from build123d import *

# Parameters (mm, degrees)
BOSS_EXTRUDE1_DEPTH     = 2
SKETCH2_R               = 1.575
BOSS_EXTRUDE2_DEPTH     = 4
SKETCH3_R               = 3.5
BOSS_EXTRUDE3_DEPTH     = 1
SKETCH4_W               = 2
SKETCH4_H               = 17
BOSS_EXTRUDE4_DEPTH     = 0.001
SKETCH5_W               = 18
SKETCH5_H               = 2
BOSS_EXTRUDE5_DEPTH     = 0.001
SKETCH6_W               = 2.001
SKETCH6_H               = 2
BOSS_EXTRUDE6_DEPTH     = 5
BOSS_EXTRUDE7_DEPTH     = 0.001
CUT_EXTRUDE1_DEPTH      = 20.519323784
SKETCH9_W               = 2.937742252
SKETCH9_H               = 8
CUT_EXTRUDE2_DEPTH      = 0.001
CUT_EXTRUDE11_START     = -0.001
SKETCH21_R              = 9.75
SKETCH21_R_2            = 3.5
CUT_EXTRUDE11_DEPTH     = 0.001
SKETCH10_W              = 32
SKETCH10_H              = 2
BOSS_EXTRUDE8_DEPTH     = 7
FILLET1_R               = 0.5
SKETCH11_R              = 0.625
BOSS_EXTRUDE9_DEPTH     = 2
SKETCH14_W              = 2
SKETCH14_H              = 2
CUT_EXTRUDE5_DEPTH      = 22.401355237
SKETCH12_R              = 0.675
CUT_EXTRUDE3_DEPTH      = 2.5
CUT_EXTRUDE6_DEPTH      = 2
FILLET2_R               = 0.5
FILLET3_R               = 0.5
FILLET4_R               = 2
CUT_EXTRUDE7_DEPTH      = 26.019992106
CUT_EXTRUDE7_DEPTH_BACK = 1
SKETCH19_R              = 0.625
CUT_EXTRUDE9_DEPTH      = 2


with BuildPart() as part:
    # Sketch1 → Boss-Extrude1 (new body)
    with BuildSketch(Plane.XY):
        Polygon((-11, 6), (-11, 11), (11, 11), (11, 6), (11, -6), (-11, -6), align=None)
    extrude(amount=BOSS_EXTRUDE1_DEPTH)

    # Sketch3 → Boss-Extrude3 (add)
    with BuildSketch(Plane(origin=(0, 0, 0), x_dir=(-1, 0, 0), z_dir=(0, 0, -1))):
        with Locations(Location((0, 0, 0), (0, 0, 180))):
            Circle(SKETCH3_R)
    extrude(amount=BOSS_EXTRUDE3_DEPTH)

    # Sketch4 → Boss-Extrude4 (add)
    with BuildSketch(Plane(origin=(0, 0, 0), x_dir=(-1, 0, 0), z_dir=(0, 0, -1))):
        with Locations((10, 2.5)):
            Rectangle(SKETCH4_W, SKETCH4_H)
        with Locations((-10, 2.5)):
            Rectangle(SKETCH4_W, SKETCH4_H)
    extrude(amount=BOSS_EXTRUDE4_DEPTH)

    # Sketch5 → Boss-Extrude5 (add)
    with BuildSketch(Plane(origin=(0, 0, 0), x_dir=(-1, 0, 0), z_dir=(0, 0, -1))):
        with Locations((0, 10)):
            Rectangle(SKETCH5_W, SKETCH5_H)
    extrude(amount=BOSS_EXTRUDE5_DEPTH)

    # Sketch6 → Boss-Extrude6 (add)
    with BuildSketch(Plane(origin=(11, 0, 0), x_dir=(0, 0, -1), z_dir=(1, 0, 0))):
        with Locations((-0.9995, -5)):
            Rectangle(SKETCH6_W, SKETCH6_H)
        with Locations((-0.9995, 5)):
            Rectangle(SKETCH6_W, SKETCH6_H)
    boss_extrude6 = extrude(amount=BOSS_EXTRUDE6_DEPTH)

    # Mirror1: Boss-Extrude6 across plane
    add(boss_extrude6.mirror(Plane(origin=(0, 0, 0), x_dir=(0, 0, 1), z_dir=(1, 0, 0))))

    # Sketch7 → Boss-Extrude7 (add)
    with BuildSketch(Plane(origin=(0, 0, -0.001), x_dir=(-1, 0, 0), z_dir=(0, 0, -1))):
        with BuildLine():
            ThreePointArc((-6.708203932, -6), (-8.407551231, -3.211398808), (-9, 0))
            Line((-9, 0), (-9, -6))
            Line((-9, -6), (-6.708203932, -6))
        make_face()
        with BuildLine():
            Line((-9, 9), (-9, 0))
            ThreePointArc((-9, 0), (-6.363961031, 6.363961031), (0, 9))
            Line((0, 9), (-9, 9))
        make_face()
    boss_extrude7 = extrude(amount=-BOSS_EXTRUDE7_DEPTH)

    # Sketch8 → Cut-Extrude1 (cut, through all)
    with BuildSketch(Plane(origin=(0, 0, -0.001), x_dir=(-1, 0, 0), z_dir=(0, 0, -1))):
        with BuildLine():
            Line((-11, 4), (-9.16515139, 4))
            ThreePointArc((-9.16515139, 4), (-10, 0), (-9.16515139, -4))
            Line((-9.16515139, -4), (-11, -4))
            Line((-11, -4), (-11, 4))
        make_face()
    cut_extrude1 = extrude(amount=-CUT_EXTRUDE1_DEPTH, mode=Mode.SUBTRACT)

    # Sketch9 → Cut-Extrude2 (cut)
    with BuildSketch(Plane(origin=(0, 0, -0.001), x_dir=(-1, 0, 0), z_dir=(0, 0, -1))):
        with Locations((-9.531128874, 0)):
            Rectangle(SKETCH9_W, SKETCH9_H)
    cut_extrude2 = extrude(amount=-CUT_EXTRUDE2_DEPTH, mode=Mode.SUBTRACT)

    # Mirror2: Boss-Extrude7, Cut-Extrude1, Cut-Extrude2 across plane
    add(boss_extrude7.mirror(Plane(origin=(0, 0, 0), x_dir=(0, 0, 1), z_dir=(1, 0, 0))))
    add(cut_extrude1.mirror(Plane(origin=(0, 0, 0), x_dir=(0, 0, 1), z_dir=(1, 0, 0))), mode=Mode.SUBTRACT)
    add(cut_extrude2.mirror(Plane(origin=(0, 0, 0), x_dir=(0, 0, 1), z_dir=(1, 0, 0))), mode=Mode.SUBTRACT)

    # Sketch21 → Cut-Extrude11 (cut)
    with BuildSketch(Plane(origin=(0, 0, -0.001), x_dir=(-1, 0, 0), z_dir=(0, 0, -1)).offset(CUT_EXTRUDE11_START)):
        Circle(SKETCH21_R)
        with Locations(Location((0, 0, 0), (0, 0, 180))):
            Circle(SKETCH21_R_2, mode=Mode.SUBTRACT)
    extrude(amount=CUT_EXTRUDE11_DEPTH, mode=Mode.SUBTRACT)

    # Sketch10 → Boss-Extrude8 (add)
    with BuildSketch(Plane.XY.offset(2)):
        with Locations((0, -5)):
            Rectangle(SKETCH10_W, SKETCH10_H)
        with Locations((0, 5)):
            Rectangle(SKETCH10_W, SKETCH10_H)
    extrude(amount=BOSS_EXTRUDE8_DEPTH)

    # Fillet1
    fillet1_edges = [part.edges().sort_by_distance(p)[0] for p in [
        (10, 0, 2),
        (-10, 0, 2),
    ]]
    fillet(fillet1_edges, radius=FILLET1_R)

    # Sketch11 → Boss-Extrude9 (add)
    with BuildSketch(Plane(origin=(0, 0, -0.001), x_dir=(-1, 0, 0), z_dir=(0, 0, -1))):
        with Locations(Location((-13, -5, 0), (0, 0, 180))):
            Circle(SKETCH11_R)
    boss_extrude9 = extrude(amount=BOSS_EXTRUDE9_DEPTH)

    # Sketch14 → Cut-Extrude5 (cut, through all)
    with BuildSketch(Plane(origin=(0, 0, -0.001), x_dir=(-1, 0, 0), z_dir=(0, 0, -1))):
        with Locations((10, 7)):
            Rectangle(SKETCH14_W, SKETCH14_H)
        with Locations((-10, 7)):
            Rectangle(SKETCH14_W, SKETCH14_H)
    extrude(amount=-CUT_EXTRUDE5_DEPTH, mode=Mode.SUBTRACT)

    # Sketch12 → Cut-Extrude3 (cut)
    with BuildSketch(Plane(origin=(0, 0, -0.001), x_dir=(-1, 0, 0), z_dir=(0, 0, -1))):
        with Locations((13, -5)):
            Circle(SKETCH12_R)
    cut_extrude3 = extrude(amount=-CUT_EXTRUDE3_DEPTH, mode=Mode.SUBTRACT)

    # Sketch16 → Cut-Extrude6 (cut)
    with BuildSketch(Plane(origin=(0, 6, 0), x_dir=(1, 0, 0), z_dir=(0, 1, 0))):
        with BuildLine():
            Line((-9, -1), (-9, -2))
            ThreePointArc((-9, -2), (-8.75, -1.5), (-9, -1))
        make_face()
    cut_extrude6 = extrude(amount=CUT_EXTRUDE6_DEPTH, mode=Mode.SUBTRACT)

    # Mirror3: Boss-Extrude9, Cut-Extrude3 across plane
    add(boss_extrude9.mirror(Plane.ZX))
    add(cut_extrude3.mirror(Plane.ZX), mode=Mode.SUBTRACT)

    # Mirror4: Cut-Extrude6 across plane
    add(cut_extrude6.mirror(Plane(origin=(0, 0, 0), x_dir=(0, 0, 1), z_dir=(1, 0, 0))), mode=Mode.SUBTRACT)

    # Fillet2
    fillet2_edges = [part.edges().sort_by_distance(p)[0] for p in [
        (12.375, -5, -0.001),
        (12.375, 5, -0.001),
    ]]
    fillet(fillet2_edges, radius=FILLET2_R)

    # Fillet3
    # the kernel refuses this fillet: 0.5 mm, written as the material it takes off along each edge
    with BuildSketch(Plane(origin=(-13, -5, -0.001), x_dir=(-1, 0, 0), z_dir=(0, -1, 0))) as fillet3_piece_1:
        with BuildLine():
            CenterArc((0.675 + FILLET3_R, -FILLET3_R), FILLET3_R, 90, 90)
            Line((0.675, -FILLET3_R), (0.675, 0))
            Line((0.675, 0), (0.675 + FILLET3_R, 0))
        make_face()
    revolve(axis=Axis((-13, -5, -0.001), (0, 0, -1)), mode=Mode.SUBTRACT)
    with BuildSketch(Plane(origin=(-13, 5, -0.001), x_dir=(-1, 0, 0), z_dir=(0, 1, 0))) as fillet3_piece_2:
        with BuildLine():
            CenterArc((0.675 + FILLET3_R, FILLET3_R), FILLET3_R, 180, 90)
            Line((0.675, FILLET3_R), (0.675, 0))
            Line((0.675, 0), (0.675 + FILLET3_R, 0))
        make_face()
    revolve(axis=Axis((-13, 5, -0.001), (0, 0, 1)), mode=Mode.SUBTRACT)

    # Fillet4
    fillet4_edges = [part.edges().sort_by_distance(p)[0] for p in [
        (16, -5, 9),
        (-16, -5, 9),
        (-16, 5, 9),
        (16, 5, 9),
    ]]
    fillet(fillet4_edges, radius=FILLET4_R)

    # Sketch17 → Cut-Extrude7 (cut, two sides: drawn at the far end of the back side and taken through both)
    with BuildSketch(Plane.XZ.offset(6).offset(-CUT_EXTRUDE7_DEPTH_BACK)):
        with BuildLine():
            Line((-16, 7), (-16, -0.001))
            Line((-16, -0.001), (-14.5, -0.001))
            Line((-14.5, -0.001), (-14.5, 7))
            ThreePointArc((-14.5, 7), (-14.353553391, 7.353553391), (-14, 7.5))
            Line((-14, 7.5), (14, 7.5))
            ThreePointArc((14, 7.5), (14.353553391, 7.353553391), (14.5, 7))
            Line((14.5, 7), (14.5, -0.001))
            Line((14.5, -0.001), (16, -0.001))
            Line((16, -0.001), (16, 7))
            ThreePointArc((16, 7), (15.414213562, 8.414213562), (14, 9))
            Line((14, 9), (-14, 9))
            ThreePointArc((-14, 9), (-15.414213562, 8.414213562), (-16, 7))
        make_face()
    extrude(amount=CUT_EXTRUDE7_DEPTH + CUT_EXTRUDE7_DEPTH_BACK, mode=Mode.SUBTRACT)

    # Sketch19 → Cut-Extrude9 (cut)
    with BuildSketch(Plane(origin=(0, 6, 0), x_dir=(1, 0, 0), z_dir=(0, 1, 0))):
        with Locations(Location((0, -2.625, 0), (0, 0, 90))):
            Circle(SKETCH19_R)
        with Locations(Location((0, -8.125, 0), (0, 0, 270))):
            Circle(SKETCH19_R)
    extrude(amount=-CUT_EXTRUDE9_DEPTH, mode=Mode.SUBTRACT)


with BuildPart() as body_2:
    # Sketch2 → Boss-Extrude2 (new body)
    with BuildSketch(Plane(origin=(0, 0, 2), x_dir=(-1, 0, 0), z_dir=(0, 0, -1))):
        Circle(SKETCH2_R)
    extrude(amount=BOSS_EXTRUDE2_DEPTH)


with BuildPart() as part_1:
    add(part.part)

    # Combine2: cut body 2
    add(body_2.part, mode=Mode.SUBTRACT)


solid = part_1.part
The listing builds one solid part. Answer for the finished solid, in the listing's coordinates (mm). A direction names the side the tool comes from. Coordinates: 2 decimals unless noted, no trailing zeros. Write each loop counter-clockwise with the first axis right and the second up, starting at its lowest first coordinate (ties: lowest second). Pieces come first, ordered by that corner, then holes. Notation, with made-up numbers: M 40.25,73.5 L 72.25,73.5 A24 ccw 72.25,91.5 Z; hole C -11.5,2 d5. An arc over 180 degrees is marked long. Put each result on its own line as item: value. Start each with the question number.
1. A cutting plane is placed at A-A on y = 0. Write down the section's boundary in (x, z) (3 decimals), then the cut area to 3 significant figures.
2. Which of the six approach directions +Z, -Z, +X, -X, +Y, -Y give full straight-line access (tool end or side, diameter ignored) to faces 4 (the flat face through (-14.5, -5.5, 3.5)), 5 (the flat face through (13, 5, -2.001)), 6 (the cylindrical face through (-0.03, 5.01, 3.25)), 7 (the cylindrical face through (13.336, 5.527, -1.23)), 8 (the flat face through (-10, -5, -0.001))?
3. A cutting plane is placed at D-D on y = 5. Count the separate pieces of the cut face and the enclosed holes in it, then the cut area to 3 significant figures.
4. Flat-ended cylindrical pins translate along their axes: P1, Ø4.5, axis at x = -0.5, z = 5, coming from the +Y side; P2, Ø0.8, axis at y = 7, z = 0.5, coming from the +X side; P3, Ø4, axis at x = -6, y = -3.5, coming from the -Z side; P4, Ø9, axis at x = -2.5, y = -1.5, coming from the +Z side. Find the tip coordinate at first contact, or state that the pin passes through.
5. For a pull along Y with two mould halves and no side action, classify faces 1 (the flat face through (9, 7, 0.5)), 2 (the flat face through (11, 9, 1)), 3 (the flat face through (0, 11, 1)) as pulls with the +Y half, pulls with the -Y half, needs draft (parallel to the pull), parting line crosses it, or undercut.
6. A cutting plane is placed at B-B on z = 5. Write down the section's boundary in (x, y).
7. Consider line 1 (Y direction, x = -6.5, z = 2.25); line 2 (X direction, y = 5, z = 1) (3 decimals); line 3 (Z direction, x = -4.5, y = -4.75). Determine where each line is inside the solid, lowest interval first. Write a range as from..to.
Resolved:
1. outline: M -10,0 L -3.5,0 L -3.5,-1 L -1.575,-1 L -1.575,2 L -9.5,2 A0.5 ccw -10,1.5 Z; M 1.575,-1 L 3.5,-1 L 3.5,0 L 10,0 L 10,1.5 A0.5 ccw 9.5,2 L 1.575,2 Z
1. area: 37.4 mm2
2. face 4: +Z, -Z, -X, -Y
2. face 5: -Z, +X, -X, +Y, -Y
2. face 6: +Y
2. face 7: -Z
2. face 8: -Z, -X, +Y, -Y
3. separate pieces: 1
3. enclosed holes: 2
3. area: 283 mm2
4. P1: stops at y = 6
4. P2: stops at x = 9
4. P3: stops at z = 0
4. P4: stops at z = 9
5. face 1: undercut
5. face 2: needs draft
5. face 3: pulls with the +Y half
6. outline: M -16,-5 L -14.5,-5 L -14.5,-6 L 14.5,-6 L 14.5,-5 L 16,-5 L 16,-4 L -16,-4 Z; M -16,4 L 16,4 L 16,6 L -16,6 Z
7. line 1: y = -6..-4, 4..6
7. line 2: x = -16..-13.675, -12.325..16
7. line 3: z = 0..9
